from build123d import *

# Parameters (mm, degrees)
SKETCH2_W              = 11
SKETCH2_H              = 116
BOSS_EXTRUDE2_DEPTH    = 109.999999964
SKETCH3_W              = 2
SKETCH3_H              = 70
CUT_EXTRUDE1_DEPTH     = 129.848748531
CUT_EXTRUDE2_DEPTH     = 7
CUT_EXTRUDE2_DRAFT     = -45
CUT_EXTRUDE3_START     = -109.999999964
CUT_EXTRUDE3_OUTLINE_R = 1.8415
CUT_EXTRUDE3_DEPTH     = 109.999999964
SKETCH7_R              = 1.8415
CUT_EXTRUDE4_DEPTH     = 25.4
CUT_EXTRUDE5_START     = -25.4
SKETCH8_R              = 1.8415
CUT_EXTRUDE5_DEPTH     = 25.4
SKETCH9_R              = 2.413
CUT_EXTRUDE6_DEPTH     = 81.684571085


# Read off the part's stored shape, not the designer's step: Cut-Extrude3
with BuildPart() as part:
    # Sketch2 → Boss-Extrude2 (new body)
    with BuildSketch(Plane.XY.offset(54.999999982)):
        with Locations((-5.5, 0)):
            Rectangle(SKETCH2_W, SKETCH2_H)
    extrude(amount=-BOSS_EXTRUDE2_DEPTH)

    # Sketch3 → Cut-Extrude1 (cut, through all)
    with BuildSketch(Plane(origin=(0, 58, 0), x_dir=(1, 0, 0), z_dir=(0, 1, 0))):
        with Locations((-1, 1.8e-08)):
            Rectangle(SKETCH3_W, SKETCH3_H)
    extrude(amount=-CUT_EXTRUDE1_DEPTH, mode=Mode.SUBTRACT)


with BuildPart() as cut_extrude2_tool:
    # Sketch5 → Cut-Extrude2 (with draft: the straight prism first)
    with BuildSketch(Plane.ZY.offset(11)):
        with BuildLine():
            Line((-44.45, 0), (-44.45, -77.05))
            Line((-44.45, -77.05), (44.45, -77.05))
            Line((44.45, -77.05), (44.45, 0))
            ThreePointArc((44.45, 0), (0, 44.45), (-44.45, 0))
        make_face()
    extrude(amount=-CUT_EXTRUDE2_DEPTH)
    # Cut-Extrude2: the draft: its side faces are tilted about the plane it starts from
    cut_extrude2_sides = [cut_extrude2_tool.faces().sort_by_distance(p)[0] for p in [
        (-7.5, -38.525, -44.45),
        (-7.5, -77.05, 0),
        (-7.5, -38.525, 44.45),
        (-7.5, 44.45, 0),
    ]]
    draft(cut_extrude2_sides, Plane.ZY.offset(11), CUT_EXTRUDE2_DRAFT)


with BuildPart() as part_1:
    add(part.part)

    # Cut-Extrude2: cut by cut_extrude2_tool
    add(cut_extrude2_tool.part, mode=Mode.SUBTRACT)

    # Cut-Extrude3 outline → Cut-Extrude3 (cut)
    with BuildSketch(Plane.XY.offset(54.999999982).offset(CUT_EXTRUDE3_START)):
        with Locations((-7.5, 0)):
            Circle(CUT_EXTRUDE3_OUTLINE_R)
    extrude(amount=CUT_EXTRUDE3_DEPTH, mode=Mode.SUBTRACT)

    # Sketch7 → Cut-Extrude4 (cut)
    with BuildSketch(Plane(origin=(0, 58, 0), x_dir=(1, 0, 0), z_dir=(0, 1, 0))):
        with Locations(Location((-5.5, -44.999999982, 0), (0, 0, 270))):
            Circle(SKETCH7_R)
        with Locations(Location((-5.5, 44.999999982, 0), (0, 0, 270))):
            Circle(SKETCH7_R)
    extrude(amount=-CUT_EXTRUDE4_DEPTH, mode=Mode.SUBTRACT)

    # Sketch8 → Cut-Extrude5 (cut)
    with BuildSketch(Plane.XZ.offset(58).offset(CUT_EXTRUDE5_START)):
        with Locations(Location((-5.5, 44.999999982, 0), (0, 0, 90))):
            Circle(SKETCH8_R)
        with Locations(Location((-5.5, -44.999999982, 0), (0, 0, 90))):
            Circle(SKETCH8_R)
    extrude(amount=CUT_EXTRUDE5_DEPTH, mode=Mode.SUBTRACT)

    # Sketch9 → Cut-Extrude6 (cut, through all)
    with BuildSketch(Plane(origin=(0, 0, 0), x_dir=(0, 0, -1), z_dir=(1, 0, 0))):
        with Locations(Location((-49.999999982, 18, 0), (0, 0, 90))):
            Circle(SKETCH9_R)
        with Locations(Location((-49.999999982, -18, 0), (0, 0, 90))):
            Circle(SKETCH9_R)
        with Locations(Location((49.999999982, -18, 0), (0, 0, 90))):
            Circle(SKETCH9_R)
        with Locations(Location((49.999999982, 18, 0), (0, 0, 90))):
            Circle(SKETCH9_R)
    extrude(amount=-CUT_EXTRUDE6_DEPTH, mode=Mode.SUBTRACT)


solid = part_1.part
Design review of the part built by this model. Coordinates are the model's own, in mm. A direction names the side the tool comes from. Coordinates: 2 decimals unless noted, no trailing zeros. Loops run counter-clockwise (first coordinate to the right, second up) from the corner with the lowest first, then second, coordinate; pieces in that order, holes last.
Item 1: For faces 5 (the flat face through (-2, 1, 0)), 6 (the cylindrical face through (-4.79, -45.12, 46.7)), 7 (the flat face through (-4, -10, -1)), 8 (the flat face through (0, -1, -45)), 9 (the flat face through (-5, 32.6, 45)), list the 3-axis set-ups (+Z, -Z, +X, -X, +Y, -Y) from which the entire face can be reached by the end or side of a thin tool; tool diameter is ignored.
Completed:
face 5: +X, +Y, -Y
face 6: -Y
face 7: -X, -Y
face 8: +Z, -Z, +X, +Y, -Y
face 9: +Y
Item 2: Add section C-C (y = -18). Write out the cut boundary in (x, z).
Completed:
outline: (-11, -55) - (0, -55) - (0, -52.41) - (-11, -52.41) - close; (-11, -47.59) - (0, -47.59) - (0, -35) - (-2, -35) - (-2, 35) - (0, 35) - (0, 47.59) - (-11, 47.59) - (-11, 44.45) - (-4, 37.45) - (-4, -37.45) - (-11, -44.45) - close; (-11, 52.41) - (0, 52.41) - (0, 55) - (-11, 55) - close
Item 3: Add section D-D (z = 0). Write out the cut boundary in (x, y), and give its area (3 significant figures).
Completed:
outline: (-11, 44.45) - (-4, 37.45) - (-4, -58) - (-2, -58) - (-2, 58) - (-11, 58) - close
area: 351 mm2
Item 4: Add section A-A (z = -50). Write out the cut boundary in (x, y).
Completed:
outline: (-11, -58) - (0, -58) - (0, -20.41) - (-11, -20.41) - close; (-11, -15.59) - (0, -15.59) - (0, 15.59) - (-11, 15.59) - close; (-11, 20.41) - (0, 20.41) - (0, 58) - (-11, 58) - close; hole circle Ø3.68 at (-7.5, 0)
Item 5: Wall thickness on L1, parallel to Z at x = -5, y = 34; L2, parallel to Z at x = -4.25, y = 18; L3, parallel to X at y = 40, z = 45: over which ranges is each line inside the solid? List them lowest first.
Completed:
L1: z = -55 to -46.77, -43.23 to -17.96, 17.96 to 43.23, 46.77 to 55
L2: z = -55 to -52.41, -47.59 to -33.13, 33.13 to 47.59, 52.41 to 55
L3: x = -11 to -7.34, -3.66 to 0
Item 6: Draft analysis for pull direction Y (two halves, no side actions). For faces 1 (the flat face through (-5, 32.6, -45)), 2 (the flat face through (-6, -32.6, -45)), 3 (the cylindrical face through (-5.423, -18.314, -47.608)), 4 (the flat face through (-5.6, 0.8, 55)), state which applies: pulls with the +Y half, pulls with the -Y half, needs draft (parallel to the pull), parting line crosses it, or undercut.
Completed:
face 1: pulls with the +Y half
face 2: pulls with the -Y half
face 3: undercut
face 4: needs draft
Item 7: Add section B-B (y = -46). Write out the cut boundary in (x, z).
Completed:
outline: (-11, -55) - (0, -55) - (0, -35) - (-2, -35) - (-2, 35) - (0, 35) - (0, 55) - (-11, 55) - (-11, 44.45) - (-4, 37.45) - (-4, -37.45) - (-11, -44.45) - close; hole circle Ø3.68 at (-5.5, -45); hole circle Ø3.68 at (-5.5, 45)
Item 8: Clearance check with flat-ended pins moving along their axes: pin 1 (2 mm diameter, centred on x = -5.5, z = 45, fed in from +Y); pin 2 (3 mm diameter, centred on y = -18, z = 50, fed in from +X); pin 3 (1.8 mm diameter, centred on x = -6, z = 45.5, fed in from -Y); pin 4 (4 mm diameter, centred on y = 2.5, z = -31, fed in from -X). State where each tip first meets the part, or that it passes through.
Completed:
pin 1: stops at y = 32.6
pin 2: passes through
pin 3: stops at y = -32.6
pin 4: stops at x = -4
